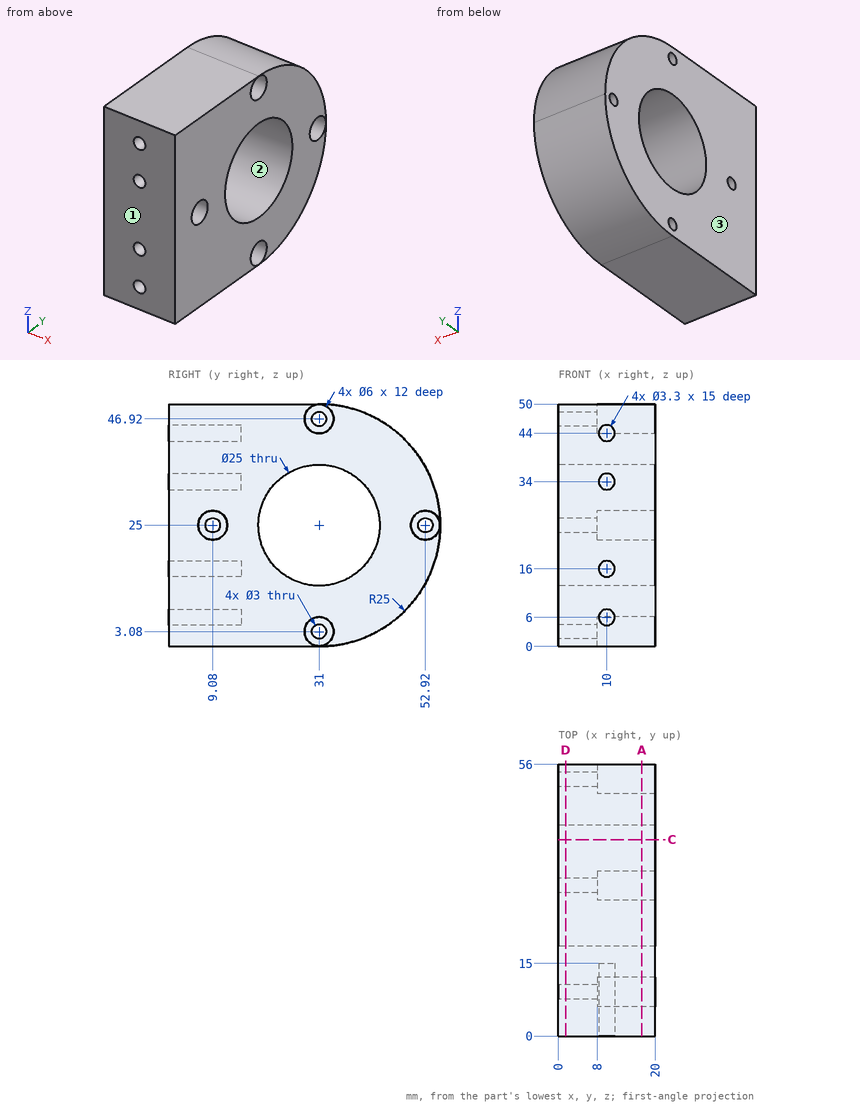
Study the drawing (mm; zero at the part's minimum x, y, z) and answer. Give positions to 0.01 mm unless a question says otherwise; leave off trailing zeros. Loops run counter-clockwise (first coordinate to the right, second up) from the corner with the lowest first, then second, coordinate; pieces in that order, holes last. Notation, with made-up numbers: (-14, 60) - (-5, 60) arc R6 cw to (-5, 69) - close; hole circle Ø1 at (79.25, 50). An arc over 180 degrees is marked (long way). One line per question, with ' | ' between items.
(1) Straight lines are drawn through the part: probe 1 along X at (y, z) = (11, 6); probe 2 along Y at (x, z) = (4.5, 26); probe 3 along X at (y, z) = (8, 22.5). For each, find the intervals that lie inside material, in ascending order.
Recorded:
probe 1: x = 0 to 8.35, 11.65 to 20 | probe 2: y = 0 to 7.96, 10.2 to 18.54, 43.46 to 51.8, 54.04 to 55.98 | probe 3: x = 0 to 8
(2) The part is cut by section A-A (x = 17.25). Write down the section's boundary in (y, z).
Recorded:
outline: (0, 0) - (31, 0) arc R25 ccw to (31, 50) - (0, 50) - close; hole circle Ø6 at (9.08, 25); hole circle Ø25 at (31, 25); hole circle Ø6 at (31, 3.08); hole circle Ø6 at (31, 46.92); hole circle Ø6 at (52.92, 25)
(3) Each of these flat-tipped pins is pushed along its axis until it touches: pin 1 Ø1 at (x, z) = (8, 41) entering from +Y (1 decimal); pin 2 Ø1.8 at (y, z) = (32, 3) entering from +X; pin 3 Ø2.5 at (x, z) = (10, 6) entering from -Y; pin 4 Ø2.5 at (y, z) = (52.92, 25) entering from +X. Where does it stop, or does it pass through?
Recorded:
pin 1: stops at y = 50.6 | pin 2: stops at x = 8 | pin 3: stops at y = 15 | pin 4: passes through
(4) The part is cut by section D-D (x = 1.5). Write down the section's boundary in (y, z).
Recorded:
outline: (0, 0) - (31, 0) arc R25 ccw to (31, 50) - (0, 50) - close; hole circle Ø3 at (9.08, 25); hole circle Ø25 at (31, 25); hole circle Ø3 at (31, 3.08); hole circle Ø3 at (31, 46.92); hole circle Ø3 at (52.92, 25)
(5) The mould has two halves that part along Y. Classify the marked faces 1, 2 and 3: +Y half, -Y half, draft (parallel to the pull), parting line (faces both ways), or undercut.
Recorded:
face 1: -Y half | face 2: undercut | face 3: draft
(6) The part is cut by section C-C (y = 40.5). Write down the section's boundary in (x, z) (1 decimal), then the cut area to 3 significant figures.
Recorded:
outline: (0, 1.9) - (20, 1.9) - (20, 16.9) - (0, 16.9) - close; (0, 33.1) - (20, 33.1) - (20, 48.1) - (0, 48.1) - close | area: 600 mm²
